from build123d import *
from OCP.BRepFilletAPI import BRepFilletAPI_MakeFillet

# Parameters (mm, degrees)
SKETCH1_W           = 30
SKETCH1_H           = 50
BOSS_EXTRUDE1_DEPTH = 3
SKETCH2_W           = 30
SKETCH2_H           = 5
BOSS_EXTRUDE2_DEPTH = 25
BOSS_EXTRUDE4_START = 3
BOSS_EXTRUDE4_DEPTH = 5
SKETCH6_W           = 5
SKETCH6_H           = 55
CUT_EXTRUDE1_DEPTH  = 35
FILLET3_R           = 5
FILLET5_R           = 3
FILLET5_R_2         = 2
FILLET6_R           = 2


with BuildPart() as part:
    # Sketch1 → Boss-Extrude1 (new body)
    with BuildSketch(Plane.XY):
        Rectangle(SKETCH1_W, SKETCH1_H)
        with BuildLine():
            Line((-11.85, 8), (-11.85, 16))
            ThreePointArc((-11.85, 16), (-10, 17.85), (-8.15, 16))
            Line((-8.15, 16), (-8.15, 8))
            ThreePointArc((-8.15, 8), (-10, 6.15), (-11.85, 8))
        make_face(mode=Mode.SUBTRACT)
        with BuildLine():
            Line((-11.864504809, 2.008993176), (-11.903242133, -5.990913037))
            ThreePointArc((-11.903242133, -5.990913037), (-10.062221828, -7.849849355), (-8.203285509, -6.008829049))
            Line((-8.203285509, -6.008829049), (-8.164548185, 1.991077164))
            ThreePointArc((-8.164548185, 1.991077164), (-10.00556849, 3.850013482), (-11.864504809, 2.008993176))
        make_face(mode=Mode.SUBTRACT)
    extrude(amount=BOSS_EXTRUDE1_DEPTH)

    # Sketch2 → Boss-Extrude2 (add)
    with BuildSketch(Plane.XY):
        with Locations((0, -27.5)):
            Rectangle(SKETCH2_W, SKETCH2_H)
    extrude(amount=BOSS_EXTRUDE2_DEPTH)

    # Sketch4 → Boss-Extrude4 (add)
    with BuildSketch(Plane.XY.offset(BOSS_EXTRUDE4_START)):
        Polygon((15, -25), (0, -25), (-15, -25), (-15, -20.5), (0, -20.5), (0, 25), (15, 25), align=None)
    extrude(amount=BOSS_EXTRUDE4_DEPTH)

    # Sketch6 → Cut-Extrude1 (cut)
    with BuildSketch(Plane.XY):
        with Locations((12.5, -2.5)):
            Rectangle(SKETCH6_W, SKETCH6_H)
    extrude(amount=CUT_EXTRUDE1_DEPTH, mode=Mode.SUBTRACT)

    # Fillet3
    fillet3_edges = [part.edges().sort_by_distance(p)[0] for p in [
        (0, 2.25, 3),
    ]]
    fillet(fillet3_edges, radius=FILLET3_R - 0.0001)  # a hair under: the kernel refuses the full size

    # Fillet5
    fillet5_edges_1 = [part.edges().sort_by_distance(p)[0] for p in [
        (-2.5, -30, 0),
        (-2.5, -30, 25),
        (10, 0, 8),
        (-2.5, 25, 0),
    ]]
    fillet5_edges_2 = [part.edges().sort_by_distance(p)[0] for p in [
        (-15, -22.75, 8),
    ]]
    fillet5 = BRepFilletAPI_MakeFillet(part.part.solid().wrapped)
    for e in fillet5_edges_1:
        fillet5.Add(FILLET5_R - 0.0001, e.wrapped)
    for e in fillet5_edges_2:
        fillet5.Add(FILLET5_R_2 - 0.0001, e.wrapped)
    add(Compound.cast(fillet5.Shape()), mode=Mode.REPLACE)  # a hair under: the kernel refuses the full size

    # Fillet6
    fillet6_edges = [part.edges().sort_by_distance(p)[0] for p in [
        (-3, -25, 8),
        (-14.414242852, -25, 7.414242852),
        (9.121349633, -25, 7.121349633),
    ]]
    fillet(fillet6_edges, radius=FILLET6_R)


solid = part.part
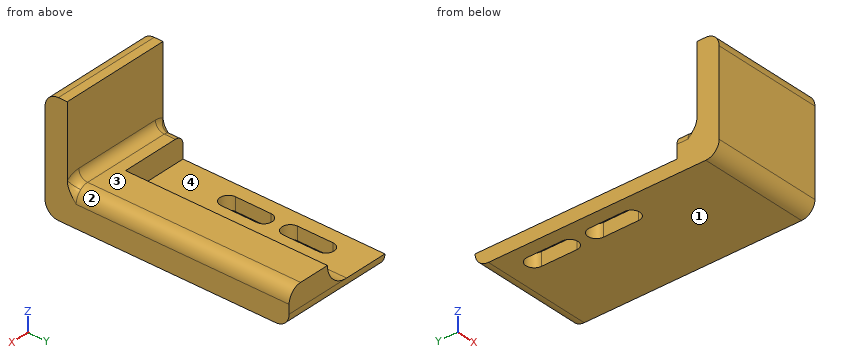
Model file for the job. Use its own axes, mm. Face numbers are marked on the shaded views. A direction names the side the tool comes from. Give positions to 0.01 mm unless a question says otherwise; leave off trailing zeros. Order: outer loops, then holes, each group sorted by start corner. A loop starts at its lowest first (then second) coordinate and runs counter-clockwise, first axis right, second up. Notation, with made-up numbers: (14, 33.25) -> (54, 33.25) arc R11 cw to (54, 50.25) -> close; hole circle Ø11 at (81.5, 43). An arc over 180 degrees is marked (long way). Use CSV: the item, a comma, the result in double quotes.
1. 3-axis set-ups, long thin cutter, end or side, ignore diameter. For the marked faces 1, 2, 3 and 4: which of +Z, -Z, +X, -X, +Y, -Y reach the whole face in a straight line?
Outcome:
face 1,"-Z, +X, -X, +Y, -Y"
face 2,"+Z, +X, +Y"
face 3,"+Z, +X, -X, +Y"
face 4,"+Z, -X, +Y"
2. Band-saw the part on C-C, the plane x = 2.25. Give the cut face in (y, z), then the cut area to 3 significant figures.
Outcome:
outline,"(-30, 3) arc R3 ccw to (-27, 0) -> (22, 0) arc R3 ccw to (25, 3) -> (25, 8) -> (-23, 8) arc R2 cw to (-25, 10) -> (-25, 25) -> (-27, 25) arc R3 ccw to (-30, 22) -> close"
area,"520 mm²"
3. Band-saw the part on D-D, the plane z = 15.75. Give the cut face in (x, y), then the cut area to 3 significant figures.
Outcome:
outline,"(-15, -30) -> (10, -30) -> (10, -25) -> (-15, -25) -> close"
area,"125 mm²"
4. Drop flat-ended pins along their axis: pin 1 (4 mm diameter, centred on x = -4, z = 6.5, fed in from +Y); pin 2 (1.5 mm diameter, centred on x = 5.5, z = 15, fed in from +Y); pin 3 (11 mm diameter, centred on x = -12, y = -8, fed in from +Z). Give the stop position or say it passes through.
Outcome:
pin 1,"y = -20.5"
pin 2,"y = -25"
pin 3,"z = 3"
5. Band-saw the part on B-B, the plane x = -10. Count the separate pieces of the cut face and the enclosed holes in it, then the cut area to 3 significant figures.
Outcome:
separate pieces,"3"
enclosed holes,"0"
area,"222 mm²"
6. Drill centre lines: line 1 along Y through (x, z) = (7.5, 13.75); line 2 along X through (y, z) = (-4, 2.75); line 3 along Z through (x, y) = (0.5, -19). Where is each one in solid material? Low to high. Write a range as from..to.
Outcome:
line 1,"-30..-25"
line 2,"-15..-11.89, -8.19..10"
line 3,"0..8"
